Read the model definition and answer for the solid it produces. Units are mm, in the model's axes. Round coordinates to 2 decimals unless told otherwise and drop trailing zeros. Write each loop counter-clockwise with the first axis right and the second up, starting at its lowest first coordinate (ties: lowest second). Pieces come first, ordered by that corner, then holes. Notation, with made-up numbers: (10.5, 82.25) - (32.5, 82.25) arc R26 ccw to (32.5, 115.25) - close; hole circle Ø10 at (13.25, -29). An arc over 180 degrees is marked (long way). One line per item, written item: value. Start each with the question number.
(1) A cutting plane is placed at A-A, the plane z = 63.5. Determine the outline of the cut face in (x, y).
(2) A cutting plane is placed at C-C, the plane y = -8.5. Determine the outline of the cut face in (x, z), plus the area to 3 significant figures.
(3) A cutting plane is placed at D-D, the plane z = 53.5. Determine the outline of the cut face in (x, y).
(4) A cutting plane is placed at B-B, the plane y = -23.5. Determine the outline of the cut face in (x, z).
(5) Find the intervals of material crossed by L1, parallel to Y at x = 127.3, z = 53.5; L2, parallel to Y at x = 127.3, z = 63.5; L3, parallel to Y at x = 126, z = 8.5, in increasing order.
from build123d import *

# Parameters (mm, degrees)
CYLINDER022_R           = 1.5
CYLINDER022_DEPTH       = 3
CYLINDER022_PITCH_ANGLE = 90
CYLINDER021_R           = 1.5
CYLINDER021_DEPTH       = 3
CYLINDER021_PITCH_ANGLE = 90
CYLINDER020_R           = 1.5
CYLINDER020_DEPTH       = 3
CYLINDER020_PITCH_ANGLE = 90
CYLINDER019_R           = 1.5
CYLINDER019_DEPTH       = 3
CYLINDER019_PITCH_ANGLE = 90
CYLINDER018_R           = 1.5
CYLINDER018_DEPTH       = 3
CYLINDER018_PITCH_ANGLE = 90
CYLINDER017_R           = 1.5
CYLINDER017_DEPTH       = 3
CYLINDER017_PITCH_ANGLE = 90
CYLINDER_R              = 1.5
CYLINDER_DEPTH          = 3
CYLINDER_PITCH_ANGLE    = 90
BOX014_W                = 111
BOX014_H                = 3
BOX014_DEPTH            = 73
BOX014_PLACEMENT_ANGLE  = 90


with BuildPart() as cylinder022:
    # Cylinder022 → Cylinder022 (new body)
    with BuildSketch(Plane.XY):
        Circle(CYLINDER022_R)
    extrude(amount=CYLINDER022_DEPTH)


with BuildPart() as cylinder022_1:
    # Cylinder022 pitch: moved
    add(cylinder022.part.rotate(Axis((0, 0, 0), (0, 1, 0)), CYLINDER022_PITCH_ANGLE))


with BuildPart() as cylinder022_2:
    # Cylinder022 placement: moved
    add(cylinder022_1.part.moved(Location((125, -8.5, 53.5))))


with BuildPart() as cylinder021:
    # Cylinder021 → Cylinder021 (new body)
    with BuildSketch(Plane.XY):
        Circle(CYLINDER021_R)
    extrude(amount=CYLINDER021_DEPTH)


with BuildPart() as cylinder021_1:
    # Cylinder021 pitch: moved
    add(cylinder021.part.rotate(Axis((0, 0, 0), (0, 1, 0)), CYLINDER021_PITCH_ANGLE))


with BuildPart() as cylinder021_2:
    # Cylinder021 placement: moved
    add(cylinder021_1.part.moved(Location((125, -23.5, 53.5))))


with BuildPart() as cylinder020:
    # Cylinder020 → Cylinder020 (new body)
    with BuildSketch(Plane.XY):
        Circle(CYLINDER020_R)
    extrude(amount=CYLINDER020_DEPTH)


with BuildPart() as cylinder020_1:
    # Cylinder020 pitch: moved
    add(cylinder020.part.rotate(Axis((0, 0, 0), (0, 1, 0)), CYLINDER020_PITCH_ANGLE))


with BuildPart() as cylinder020_2:
    # Cylinder020 placement: moved
    add(cylinder020_1.part.moved(Location((125, -8.5, 63.5))))


with BuildPart() as cylinder019:
    # Cylinder019 → Cylinder019 (new body)
    with BuildSketch(Plane.XY):
        Circle(CYLINDER019_R)
    extrude(amount=CYLINDER019_DEPTH)


with BuildPart() as cylinder019_1:
    # Cylinder019 pitch: moved
    add(cylinder019.part.rotate(Axis((0, 0, 0), (0, 1, 0)), CYLINDER019_PITCH_ANGLE))


with BuildPart() as cylinder019_2:
    # Cylinder019 placement: moved
    add(cylinder019_1.part.moved(Location((125, -23.5, -0.5))))


with BuildPart() as cylinder018:
    # Cylinder018 → Cylinder018 (new body)
    with BuildSketch(Plane.XY):
        Circle(CYLINDER018_R)
    extrude(amount=CYLINDER018_DEPTH)


with BuildPart() as cylinder018_1:
    # Cylinder018 pitch: moved
    add(cylinder018.part.rotate(Axis((0, 0, 0), (0, 1, 0)), CYLINDER018_PITCH_ANGLE))


with BuildPart() as cylinder018_2:
    # Cylinder018 placement: moved
    add(cylinder018_1.part.moved(Location((125, -23.5, 9.5))))


with BuildPart() as cylinder017:
    # Cylinder017 → Cylinder017 (new body)
    with BuildSketch(Plane.XY):
        Circle(CYLINDER017_R)
    extrude(amount=CYLINDER017_DEPTH)


with BuildPart() as cylinder017_1:
    # Cylinder017 pitch: moved
    add(cylinder017.part.rotate(Axis((0, 0, 0), (0, 1, 0)), CYLINDER017_PITCH_ANGLE))


with BuildPart() as cylinder017_2:
    # Cylinder017 placement: moved
    add(cylinder017_1.part.moved(Location((125, -8.5, 9.5))))


with BuildPart() as cylinder:
    # Cylinder → Cylinder (new body)
    with BuildSketch(Plane.XY):
        Circle(CYLINDER_R)
    extrude(amount=CYLINDER_DEPTH)


with BuildPart() as cylinder_1:
    # Cylinder pitch: moved
    add(cylinder.part.rotate(Axis((0, 0, 0), (0, 1, 0)), CYLINDER_PITCH_ANGLE))


with BuildPart() as cylinder_2:
    # Cylinder placement: moved
    add(cylinder_1.part.moved(Location((125, -8.5, -0.5))))


with BuildPart() as cut032:
    # Box014 → Box014 (new body)
    with BuildSketch(Plane.XY):
        with Locations((55.5, 1.5)):
            Rectangle(BOX014_W, BOX014_H)
    extrude(amount=BOX014_DEPTH)


with BuildPart() as cut032_1:
    # Box014 placement: moved
    add(cut032.part.moved(Location((128, -27, -5))).rotate(Axis((128, -27, -5), (0, 0, 1)), BOX014_PLACEMENT_ANGLE))

    # Cut026: cut Cylinder
    add(cylinder_2.part, mode=Mode.SUBTRACT)

    # Cut027: cut Cylinder017
    add(cylinder017_2.part, mode=Mode.SUBTRACT)

    # Cut028: cut Cylinder018
    add(cylinder018_2.part, mode=Mode.SUBTRACT)

    # Cut029: cut Cylinder019
    add(cylinder019_2.part, mode=Mode.SUBTRACT)

    # Cut030: cut Cylinder020
    add(cylinder020_2.part, mode=Mode.SUBTRACT)

    # Cut031: cut Cylinder021
    add(cylinder021_2.part, mode=Mode.SUBTRACT)

    # Cut032: cut Cylinder022
    add(cylinder022_2.part, mode=Mode.SUBTRACT)


solid = cut032_1.part
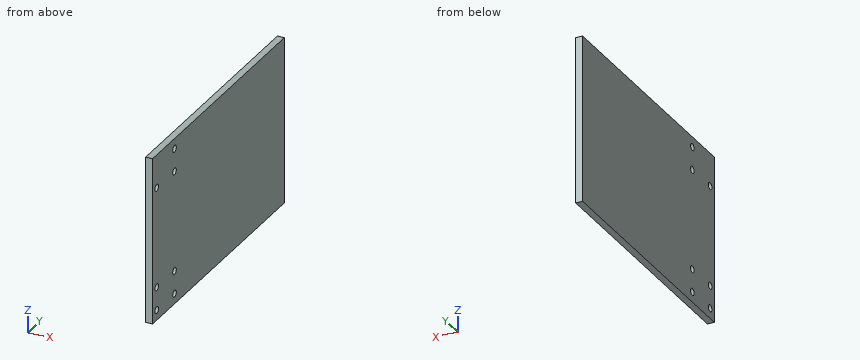
Here are the results:
1. outline: (125, -27) - (128, -27) - (128, -10) - (125, -10) - close; (125, -7) - (128, -7) - (128, 84) - (125, 84) - close
2. outline: (125, -5) - (128, -5) - (128, -2) - (125, -2) - close; (125, 1) - (128, 1) - (128, 8) - (125, 8) - close; (125, 11) - (128, 11) - (128, 52) - (125, 52) - close; (125, 55) - (128, 55) - (128, 62) - (125, 62) - close; (125, 65) - (128, 65) - (128, 68) - (125, 68) - close
2. area: 183 mm²
3. outline: (125, -27) - (128, -27) - (128, -25) - (125, -25) - close; (125, -22) - (128, -22) - (128, -10) - (125, -10) - close; (125, -7) - (128, -7) - (128, 84) - (125, 84) - close
4. outline: (125, -5) - (128, -5) - (128, -2) - (125, -2) - close; (125, 1) - (128, 1) - (128, 8) - (125, 8) - close; (125, 11) - (128, 11) - (128, 52) - (125, 52) - close; (125, 55) - (128, 55) - (128, 68) - (125, 68) - close
5. L1: -27 to -25, -22 to -10, -7 to 84
5. L2: -27 to -10, -7 to 84
5. L3: -27 to -24.62, -22.38 to -9.62, -7.38 to 84
